CAD build for the part. Positions are in the model's coordinates, mm. Face numbers are marked on the shaded views. Give positions to 0.01 mm unless a question says otherwise; leave off trailing zeros. Write each loop counter-clockwise with the first axis right and the second up, starting at its lowest first coordinate (ties: lowest second). Pieces come first, ordered by that corner, then holes. Notation, with made-up numbers: (-38, -17) - (16, -17) arc R19 ccw to (16, -10) - close; hole circle Ø3 at (0.25, -6.75). An arc over 180 degrees is marked (long way). Answer as a JSON object with one key per item and string values.
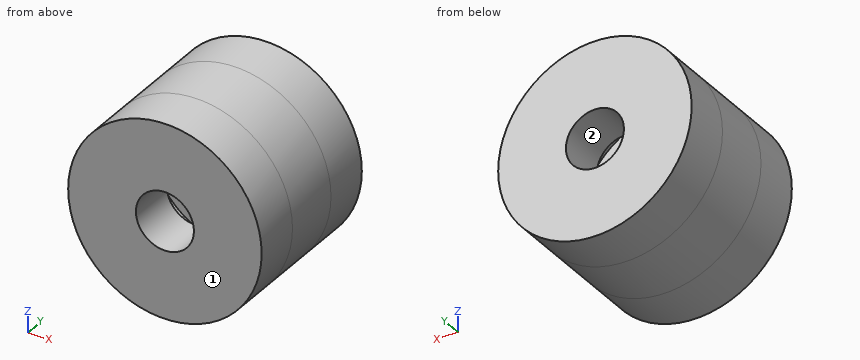
from build123d import *

# Parameters (mm, degrees)
F0_R     = 25.4
F0_R_2   = 7.62
F1_DEPTH = 12.7
F2_R     = 25.4
F3_DEPTH = 15.875
F4_R     = 25.4
F4_R_2   = 7.62
F5_DEPTH = 12.7


with BuildPart() as f1:
    # F0 (on Front) → F1 (new body)
    with BuildSketch(Plane.XZ):
        Circle(F0_R)
        Circle(F0_R_2, mode=Mode.SUBTRACT)
    extrude(amount=F1_DEPTH)

    # F2 (on face) → F3 (join)
    with BuildSketch(Plane(origin=(0, 0, 0), x_dir=(-1, 0, 0), z_dir=(0, 1, 0))):
        Circle(F2_R)
        with BuildLine():
            ThreePointArc((1.905, 22.143207), (0, -22.225), (-1.905, 22.143207))
            ThreePointArc((-1.905, 22.143207), (0, 22.491378), (1.905, 22.143207))
        make_face(mode=Mode.SUBTRACT)
    extrude(amount=F3_DEPTH)

    # F4 (on face) → F5 (join)
    with BuildSketch(Plane(origin=(0, 15.875, 0), x_dir=(-1, 0, 0), z_dir=(0, 1, 0))):
        Circle(F4_R)
        Circle(F4_R_2, mode=Mode.SUBTRACT)
    extrude(amount=F5_DEPTH)


solid = f1.part
(1) Saw through at D-D, the plane z = -10.5. Give the cut face in (x, y) (3 decimals).
Answer key:
{"outline": "(-23.128, -12.7) - (23.128, -12.7) - (23.128, 28.575) - (-23.128, 28.575) - close; hole (-19.588, 0) - (19.588, 0) - (19.588, 15.875) - (-19.588, 15.875) - close"}
(2) Pull direction X, two halves, no side cores. Call the marked faces 1 and 2: pulls with the +X half, pulls with the -X half, needs draft (parallel to the pull), parting line crosses it, or undercut.
Answer key:
{"face 1": "needs draft", "face 2": "undercut"}
(3) Saw through at C-C, the plane x = 20.5. Give the cut face in (y, z) (3 decimals), and give its area (3 significant figures).
Answer key:
{"outline": "(-12.7, -14.997) - (28.575, -14.997) - (28.575, 14.997) - (-12.7, 14.997) - close; hole (0, -8.585) - (15.875, -8.585) - (15.875, 8.585) - (0, 8.585) - close", "area": "965 mm²"}
(4) Saw through at A-A, the plane z = 0. Give the cut face in (x, y) (3 decimals), and give its area (3 significant figures).
Answer key:
{"outline": "(-25.4, -12.7) - (-7.62, -12.7) - (-7.62, 0) - (-22.225, 0) - (-22.225, 15.875) - (-7.62, 15.875) - (-7.62, 28.575) - (-25.4, 28.575) - close; (7.62, -12.7) - (25.4, -12.7) - (25.4, 28.575) - (7.62, 28.575) - (7.62, 15.875) - (22.225, 15.875) - (22.225, 0) - (7.62, 0) - close", "area": "1,000 mm²"}
(5) Flat gauge pins, fed straight in: P1, Ø8, axis at y = 5.5, z = -12, coming from the -X side; P2, Ø9, axis at x = 0, z = 0, coming from the +Y side; P3, Ø3, axis at y = -4, z = -12.5, coming from the +X side; P4, Ø17.5, axis at x = 0, z = 0, coming from the -Y side. Where does each tip first touch, or does it go through?
Answer key:
{"P1": "stops at x = -24.11", "P2": "passes through", "P3": "stops at x = 22.89", "P4": "stops at y = -12.7"}
(6) Saw through at B-B, the plane x = 0. Give the cut face in (y, z) (3 decimals), and give its area (4 significant figures).
Answer key:
{"outline": "(-12.7, -25.4) - (28.575, -25.4) - (28.575, -7.62) - (15.875, -7.62) - (15.875, -22.225) - (0, -22.225) - (0, -7.62) - (-12.7, -7.62) - close; (-12.7, 7.62) - (0, 7.62) - (0, 22.491) - (15.875, 22.491) - (15.875, 7.62) - (28.575, 7.62) - (28.575, 25.4) - (-12.7, 25.4) - close", "area": "1,000 mm²"}
(7) Probe L1, parallel to Z at x = 0, y = 25; L2, parallel to Z at x = 0, y = 9 (3 decimals); L3, parallel to Y at x = -16, z = -14 (3 decimals). List the from-to ranges inside material, lowest first. Write a range as [from, to].
Answer key:
{"L1": "z = [-25.4, -7.62], [7.62, 25.4]", "L2": "z = [-25.4, -22.225], [22.491, 25.4]", "L3": "y = [-12.7, 0], [15.875, 28.575]"}
